Read the model definition and answer for the solid it produces. Units are mm, in the model's axes. Face numbers are marked on the shaded views. A direction names the side the tool comes from. Coordinates: 2 decimals unless noted, no trailing zeros. Order: outer loops, then holes, each group sorted by start corner. A loop starts at its lowest first (then second) coordinate and runs counter-clockwise, first axis right, second up. Notation, with made-up numbers: (-35.75, 42.5) -> (-30.75, 42.5) arc R22 cw to (-30.75, 58.5) -> close; hole circle Ø2 at (69, -0.75). An arc over 180 degrees is marked (long way). Answer as a JSON object with one key per item and string values. Group by question number.
1) Consider L1, parallel to Y at x = 30, z = 1; L2, parallel to Z at x = -30, y = 10.9; L3, parallel to Z at x = 15, y = 11.45. Determine where each line is inside the solid, lowest interval first.
2) A tool of negligible diameter and unlimited length cuts with its end or side. For the marked faces 1 and 2, from which of +Z, -Z, +X, -X, +Y, -Y can it reach the whole face along a straight path? Write none if from no direction.
3) Section A-A on x = 15 is taken. Determine the outline of the cut face in (y, z), and give its area (3 significant figures).
4) Section B-B on x = 30 is taken. Determine the outline of the cut face in (y, z), and give its area (3 significant figures).
5) Given pin 1 (17 mm diameter, centred on x = -9.5, z = 23.5, fed in from -Y); pin 2 (10 mm diameter, centred on x = 23, y = -6.5, fed in from +Z); pin 3 (5 mm diameter, centred on x = 10, y = 0, fed in from -Z); pin 4 (6 mm diameter, centred on y = 10, z = 47, fed in from -X), each flat-ended and moving along its own axis, determine where each tip first touches the part or whether it passes through.
6) Section D-D on y = -4.5 is taken. Determine the outline of the cut face in (x, z).
7) Section C-C on z = 50 is taken. Determine the outline of the cut face in (x, y).
from build123d import *

# Parameters (mm, degrees)
SKETCH1_W                      = 80
SKETCH1_H                      = 20
SKETCH1_R                      = 2.7
BOSS_EXTRUDE1_DEPTH            = 3
BOSS_EXTRUDE2_DEPTH            = 20
SKETCH2_W                      = 80
SKETCH2_H                      = 3
BOSS_EXTRUDE3_DEPTH            = 40
SKETCH3_R                      = 4.75
BOSS_EXTRUDE5_DEPTH            = 4
BOSS_EXTRUDE5_TAPER            = 30
CUT_EXTRUDE2_REACH             = 25
SKETCH3_6_R                    = 1
SKETCH3_6_R_2                  = 2.7
CUT_EXTRUDE2_DIRECTION_2_REACH = 6
CUT_EXTRUDE3_DEPTH             = 57
CUT_EXTRUDE4_DEPTH             = 20
CUT_EXTRUDE5_DEPTH             = 80


with BuildPart() as part:
    # Sketch1 → Boss-Extrude1 (new body)
    with BuildSketch(Plane.XY):
        Rectangle(SKETCH1_W, SKETCH1_H)
        with Locations((-30, 0)):
            Circle(SKETCH1_R, mode=Mode.SUBTRACT)
        with Locations((-10, 0)):
            Circle(SKETCH1_R, mode=Mode.SUBTRACT)
        with Locations((10, 0)):
            Circle(SKETCH1_R, mode=Mode.SUBTRACT)
        with Locations((30, 0)):
            Circle(SKETCH1_R, mode=Mode.SUBTRACT)
    extrude(amount=BOSS_EXTRUDE1_DEPTH)

    # Sketch1<3> → Boss-Extrude2 (add)
    with BuildSketch(Plane.XY):
        Polygon((40, 13), (40, 10), (-40, 10), (-40, -10), (-43, -10), (-43, 13), align=None)
    extrude(amount=BOSS_EXTRUDE2_DEPTH)

    # Sketch2 → Boss-Extrude3 (add)
    with BuildSketch(Plane.XY.offset(20)):
        with Locations((0, 11.5)):
            Rectangle(SKETCH2_W, SKETCH2_H)
    extrude(amount=BOSS_EXTRUDE3_DEPTH)

    # Sketch3 → Boss-Extrude5 (add)
    with BuildSketch(Plane.XZ.offset(-13)):
        with Locations((15, 41.5)):
            Circle(SKETCH3_R)
        with Locations((5, 41.5)):
            Circle(SKETCH3_R)
        with Locations((-5, 41.5)):
            Circle(SKETCH3_R)
        with Locations((-15, 41.5)):
            Circle(SKETCH3_R)
    extrude(amount=-BOSS_EXTRUDE5_DEPTH, taper=BOSS_EXTRUDE5_TAPER)

    # Cut-Extrude2: up to this face of the body (flat: up to its plane)
    cut_extrude2_end = Plane(part.part.faces().sort_by_distance((0, 10, 31.5))[0])
    # Sketch3<6> → Cut-Extrude2 (cut, up to the picked face)
    with BuildSketch(Plane.XZ.offset(-13), mode=Mode.PRIVATE) as cut_extrude2_sk1:
        with Locations((-15, 41.5)):
            Circle(SKETCH3_6_R)
    cut_extrude2_tool1 = split(extrude(cut_extrude2_sk1.sketch, amount=CUT_EXTRUDE2_REACH, mode=Mode.PRIVATE), bisect_by=cut_extrude2_end, keep=Keep.BOTH, mode=Mode.PRIVATE)
    add(cut_extrude2_tool1.solids().sort_by_distance((-15, 13, 41.5))[0], mode=Mode.SUBTRACT)
    # Sketch3<6> → Cut-Extrude2 (cut, up to the picked face)
    with BuildSketch(Plane.XZ.offset(-13), mode=Mode.PRIVATE) as cut_extrude2_sk2:
        with Locations((5, 41.5)):
            Circle(SKETCH3_6_R)
    cut_extrude2_tool2 = split(extrude(cut_extrude2_sk2.sketch, amount=CUT_EXTRUDE2_REACH, mode=Mode.PRIVATE), bisect_by=cut_extrude2_end, keep=Keep.BOTH, mode=Mode.PRIVATE)
    add(cut_extrude2_tool2.solids().sort_by_distance((5, 13, 41.5))[0], mode=Mode.SUBTRACT)
    # Sketch3<6> → Cut-Extrude2 (cut, up to the picked face)
    with BuildSketch(Plane.XZ.offset(-13), mode=Mode.PRIVATE) as cut_extrude2_sk3:
        with Locations((-30, 50)):
            Circle(SKETCH3_6_R_2)
    cut_extrude2_tool3 = split(extrude(cut_extrude2_sk3.sketch, amount=CUT_EXTRUDE2_REACH, mode=Mode.PRIVATE), bisect_by=cut_extrude2_end, keep=Keep.BOTH, mode=Mode.PRIVATE)
    add(cut_extrude2_tool3.solids().sort_by_distance((-30, 13, 50))[0], mode=Mode.SUBTRACT)
    # Sketch3<6> → Cut-Extrude2 (cut, up to the picked face)
    with BuildSketch(Plane.XZ.offset(-13), mode=Mode.PRIVATE) as cut_extrude2_sk4:
        with Locations((30, 50)):
            Circle(SKETCH3_6_R_2)
    cut_extrude2_tool4 = split(extrude(cut_extrude2_sk4.sketch, amount=CUT_EXTRUDE2_REACH, mode=Mode.PRIVATE), bisect_by=cut_extrude2_end, keep=Keep.BOTH, mode=Mode.PRIVATE)
    add(cut_extrude2_tool4.solids().sort_by_distance((30, 13, 50))[0], mode=Mode.SUBTRACT)
    # Sketch3<6> → Cut-Extrude2 (cut, up to the picked face)
    with BuildSketch(Plane.XZ.offset(-13), mode=Mode.PRIVATE) as cut_extrude2_sk5:
        with Locations((15, 41.5)):
            Circle(SKETCH3_6_R)
    cut_extrude2_tool5 = split(extrude(cut_extrude2_sk5.sketch, amount=CUT_EXTRUDE2_REACH, mode=Mode.PRIVATE), bisect_by=cut_extrude2_end, keep=Keep.BOTH, mode=Mode.PRIVATE)
    add(cut_extrude2_tool5.solids().sort_by_distance((15, 13, 41.5))[0], mode=Mode.SUBTRACT)
    # Sketch3<6> → Cut-Extrude2 (cut, up to the picked face)
    with BuildSketch(Plane.XZ.offset(-13), mode=Mode.PRIVATE) as cut_extrude2_sk6:
        with Locations((-5, 41.5)):
            Circle(SKETCH3_6_R)
    cut_extrude2_tool6 = split(extrude(cut_extrude2_sk6.sketch, amount=CUT_EXTRUDE2_REACH, mode=Mode.PRIVATE), bisect_by=cut_extrude2_end, keep=Keep.BOTH, mode=Mode.PRIVATE)
    add(cut_extrude2_tool6.solids().sort_by_distance((-5, 13, 41.5))[0], mode=Mode.SUBTRACT)

    # Cut-Extrude2 direction 2: up to this face of the body (flat: up to its plane)
    cut_extrude2_direction_2_end = Plane(part.part.faces().sort_by_distance((-15, 17, 41.5))[0])
    # Sketch3<6> → Cut-Extrude2 direction 2 (cut, up to the picked face)
    with BuildSketch(Plane.XZ.offset(-13), mode=Mode.PRIVATE) as cut_extrude2_direction_2_sk1:
        with Locations((-15, 41.5)):
            Circle(SKETCH3_6_R)
    cut_extrude2_direction_2_tool1 = split(extrude(cut_extrude2_direction_2_sk1.sketch, amount=-CUT_EXTRUDE2_DIRECTION_2_REACH, mode=Mode.PRIVATE), bisect_by=cut_extrude2_direction_2_end, keep=Keep.BOTH, mode=Mode.PRIVATE)
    add(cut_extrude2_direction_2_tool1.solids().sort_by_distance((-15, 13, 41.5))[0], mode=Mode.SUBTRACT)
    # Sketch3<6> → Cut-Extrude2 direction 2 (cut, up to the picked face)
    with BuildSketch(Plane.XZ.offset(-13), mode=Mode.PRIVATE) as cut_extrude2_direction_2_sk2:
        with Locations((5, 41.5)):
            Circle(SKETCH3_6_R)
    cut_extrude2_direction_2_tool2 = split(extrude(cut_extrude2_direction_2_sk2.sketch, amount=-CUT_EXTRUDE2_DIRECTION_2_REACH, mode=Mode.PRIVATE), bisect_by=cut_extrude2_direction_2_end, keep=Keep.BOTH, mode=Mode.PRIVATE)
    add(cut_extrude2_direction_2_tool2.solids().sort_by_distance((5, 13, 41.5))[0], mode=Mode.SUBTRACT)
    # Sketch3<6> → Cut-Extrude2 direction 2 (cut, up to the picked face)
    with BuildSketch(Plane.XZ.offset(-13), mode=Mode.PRIVATE) as cut_extrude2_direction_2_sk3:
        with Locations((-30, 50)):
            Circle(SKETCH3_6_R_2)
    cut_extrude2_direction_2_tool3 = split(extrude(cut_extrude2_direction_2_sk3.sketch, amount=-CUT_EXTRUDE2_DIRECTION_2_REACH, mode=Mode.PRIVATE), bisect_by=cut_extrude2_direction_2_end, keep=Keep.BOTH, mode=Mode.PRIVATE)
    add(cut_extrude2_direction_2_tool3.solids().sort_by_distance((-30, 13, 50))[0], mode=Mode.SUBTRACT)
    # Sketch3<6> → Cut-Extrude2 direction 2 (cut, up to the picked face)
    with BuildSketch(Plane.XZ.offset(-13), mode=Mode.PRIVATE) as cut_extrude2_direction_2_sk4:
        with Locations((30, 50)):
            Circle(SKETCH3_6_R_2)
    cut_extrude2_direction_2_tool4 = split(extrude(cut_extrude2_direction_2_sk4.sketch, amount=-CUT_EXTRUDE2_DIRECTION_2_REACH, mode=Mode.PRIVATE), bisect_by=cut_extrude2_direction_2_end, keep=Keep.BOTH, mode=Mode.PRIVATE)
    add(cut_extrude2_direction_2_tool4.solids().sort_by_distance((30, 13, 50))[0], mode=Mode.SUBTRACT)
    # Sketch3<6> → Cut-Extrude2 direction 2 (cut, up to the picked face)
    with BuildSketch(Plane.XZ.offset(-13), mode=Mode.PRIVATE) as cut_extrude2_direction_2_sk5:
        with Locations((15, 41.5)):
            Circle(SKETCH3_6_R)
    cut_extrude2_direction_2_tool5 = split(extrude(cut_extrude2_direction_2_sk5.sketch, amount=-CUT_EXTRUDE2_DIRECTION_2_REACH, mode=Mode.PRIVATE), bisect_by=cut_extrude2_direction_2_end, keep=Keep.BOTH, mode=Mode.PRIVATE)
    add(cut_extrude2_direction_2_tool5.solids().sort_by_distance((15, 13, 41.5))[0], mode=Mode.SUBTRACT)
    # Sketch3<6> → Cut-Extrude2 direction 2 (cut, up to the picked face)
    with BuildSketch(Plane.XZ.offset(-13), mode=Mode.PRIVATE) as cut_extrude2_direction_2_sk6:
        with Locations((-5, 41.5)):
            Circle(SKETCH3_6_R)
    cut_extrude2_direction_2_tool6 = split(extrude(cut_extrude2_direction_2_sk6.sketch, amount=-CUT_EXTRUDE2_DIRECTION_2_REACH, mode=Mode.PRIVATE), bisect_by=cut_extrude2_direction_2_end, keep=Keep.BOTH, mode=Mode.PRIVATE)
    add(cut_extrude2_direction_2_tool6.solids().sort_by_distance((-5, 13, 41.5))[0], mode=Mode.SUBTRACT)

    # Sketch4 → Cut-Extrude3 (cut)
    with BuildSketch(Plane.XY.offset(3)):
        with BuildLine():
            Line((-39.469669914, 10.530330086), (-39.085786438, 10.146446609))
            ThreePointArc((-39.085786438, 10.146446609), (-38.923574763, 10.038060234), (-38.732233047, 10))
            Line((-38.732233047, 10), (-40, 8.732233047))
            ThreePointArc((-40, 8.732233047), (-40.038060234, 8.923574763), (-40.146446609, 9.085786438))
            Line((-40.146446609, 9.085786438), (-40.530330086, 9.469669914))
            ThreePointArc((-40.530330086, 9.469669914), (-40.530330086, 10.530330086), (-39.469669914, 10.530330086))
        make_face()
    extrude(amount=CUT_EXTRUDE3_DEPTH, mode=Mode.SUBTRACT)

    # Sketch5 → Cut-Extrude4 (cut)
    with BuildSketch(Plane.XZ.offset(10)):
        Polygon((-40, 3), (-40.5, 3), (-40, 4), align=None)
    extrude(amount=-CUT_EXTRUDE4_DEPTH, mode=Mode.SUBTRACT)

    # Sketch6 → Cut-Extrude5 (cut)
    with BuildSketch(Plane(origin=(40, 0, 0), x_dir=(0, 0, -1), z_dir=(1, 0, 0))):
        Polygon((-3, 10), (-3, 10.5), (-4, 10), align=None)
    extrude(amount=-CUT_EXTRUDE5_DEPTH, mode=Mode.SUBTRACT)


solid = part.part
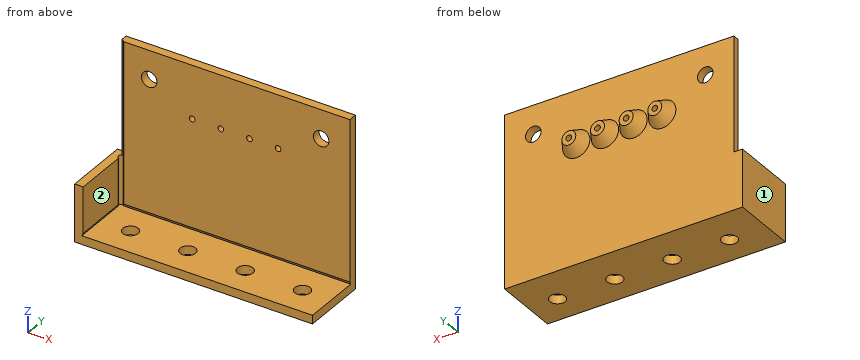
Worked answers:
{
 "1": {"L1": "y = -10 to -2.7, 2.7 to 13", "L2": "z = 0 to 47.3, 52.7 to 60", "L3": "z = 0 to 40.5, 42.5 to 60"},
 "2": {"face 1": "+Z, -Z, -X, +Y, -Y", "face 2": "+Z, +X, -Y"},
 "3": {"outline": "(-10, 0) -> (13, 0) -> (13, 36.75) -> (17, 39.06) -> (17, 40.5) -> (10, 40.5) -> (10, 4) -> (10.5, 3) -> (-10, 3) -> close; (10, 42.5) -> (17, 42.5) -> (17, 43.94) -> (13, 46.25) -> (13, 60) -> (10, 60) -> close", "area": "255 mm²"},
 "4": {"outline": "(-10, 0) -> (-2.7, 0) -> (-2.7, 3) -> (-10, 3) -> close; (2.7, 0) -> (13, 0) -> (13, 47.3) -> (10, 47.3) -> (10, 4) -> (10.5, 3) -> (2.7, 3) -> close; (10, 52.7) -> (13, 52.7) -> (13, 60) -> (10, 60) -> close", "area": "207 mm²"},
 "5": {"pin 1": "stops at y = 10", "pin 2": "stops at z = 3", "pin 3": "passes through", "pin 4": "stops at x = -40"},
 "6": {"outline": "(-43, 0) -> (40, 0) -> (40, 3) -> (-40.5, 3) -> (-40, 4) -> (-40, 20) -> (-43, 20) -> close"},
 "7": {"outline": "(-40, 10.75) arc R0.75 cw to (-39.47, 10.53) -> (-39.09, 10.15) arc R0.5 ccw to (-38.73, 10) -> (-32.7, 10) -> (-32.7, 13) -> (-40, 13) -> close; (-27.3, 10) -> (27.3, 10) -> (27.3, 13) -> (-27.3, 13) -> close; (32.7, 10) -> (40, 10) -> (40, 13) -> (32.7, 13) -> close"}
}
